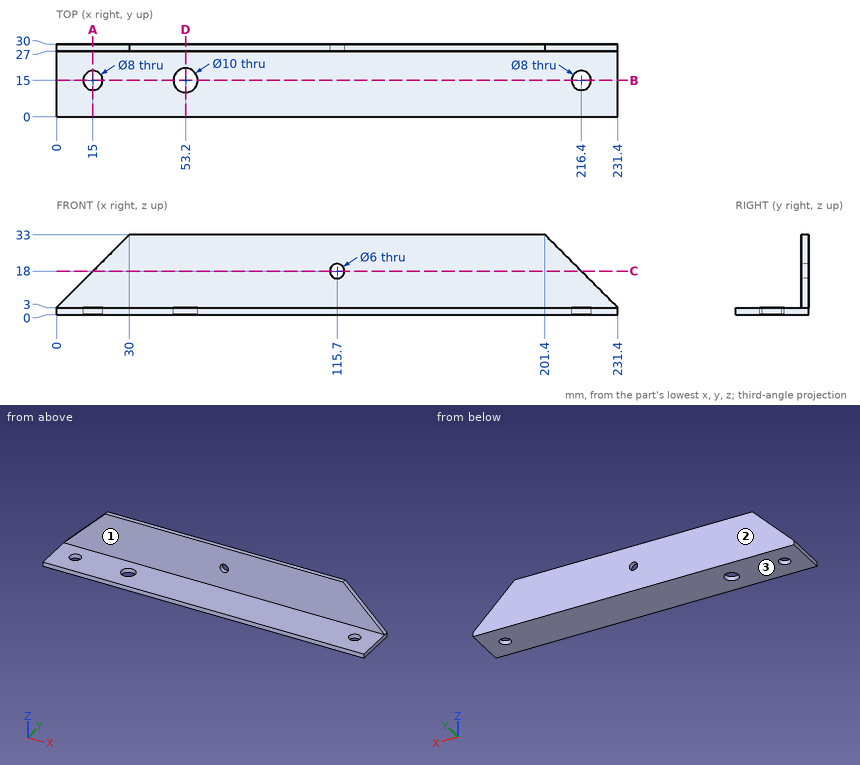
Verification items for this drawing (mm, ordinates from the low corner). Give positions to 0.01 mm unless a question says otherwise; leave off trailing zeros. Write each loop counter-clockwise with the first axis right and the second up, starting at its lowest first coordinate (ties: lowest second). Pieces come first, ordered by that corner, then holes. Notation, with made-up numbers: (27, -25) - (79, -25) arc R13 cw to (79, -18) - close; hole circle Ø10 at (74, 27). An arc over 180 degrees is marked (long way). Answer as a JSON object with one key per item and string values. Group by question number.
1) Thickness scan on probe 1 along Z at (x, y) = (115.7, 28.3); probe 2 along Y at (x, z) = (15, 0.75); probe 3 along Z at (x, y) = (217.5, 20). Record the ranges inside material, lowest first. Write a range as from..to.
2) Depth check by flat-ended pin: P1, Ø12, axis at y = 22.5, z = 10.5, coming from the -X side; P2, Ø2, axis at x = 95.5, y = 13, coming from the +Z side. Enter the tip coordinate at first touch or a pass-through.
3) Sectioned sample at B-B (y = 15). Record the cut outline in (x, z).
4) Release check for a two-part mould opening along Y. For the marked faces 1, 2 and 3 record: pulls with the +Y half, pulls with the -Y half, needs draft (parallel to the pull), parting line crosses it, or undercut.
5) Sectioned sample at D-D (x = 53.2). Record the cut outline in (y, z).
6) Sectioned sample at C-C (z = 18). Record the cut outline in (x, y).
7) Sectioned sample at A-A (x = 15). Record the cut outline in (y, z), then the cut area to 3 significant figures.
Geometry results:
{
 "1": {"probe 1": "z = 0..15, 21..33", "probe 2": "y = 0..11, 19..30", "probe 3": "z = 0..3"},
 "2": {"P1": "stops at x = 3.53", "P2": "stops at z = 3"},
 "3": {"outline": "(0, 0) - (11, 0) - (11, 3) - (0, 3) - close; (19, 0) - (48.2, 0) - (48.2, 3) - (19, 3) - close; (58.2, 0) - (212.4, 0) - (212.4, 3) - (58.2, 3) - close; (220.4, 0) - (231.4, 0) - (231.4, 3) - (220.4, 3) - close"},
 "4": {"face 1": "pulls with the -Y half", "face 2": "pulls with the +Y half", "face 3": "needs draft"},
 "5": {"outline": "(0, 0) - (10, 0) - (10, 3) - (0, 3) - close; (20, 0) - (30, 0) - (30, 33) - (27, 33) - (27, 3) - (20, 3) - close"},
 "6": {"outline": "(15, 27) - (112.7, 27) - (112.7, 30) - (15, 30) - close; (118.7, 27) - (216.4, 27) - (216.4, 30) - (118.7, 30) - close"},
 "7": {"outline": "(0, 0) - (11, 0) - (11, 3) - (0, 3) - close; (19, 0) - (30, 0) - (30, 18) - (27, 18) - (27, 3) - (19, 3) - close", "area": "111 mm^2"}
}
